from build123d import *

# Parameters (mm, degrees)
CROQUIS1_W               = 63
CROQUIS1_H               = 63
CROQUIS1_R               = 2
CROQUIS1_R_2             = 1.5
CROQUIS1_W_2             = 3
CROQUIS1_H_2             = 12
SALIENTE_EXTRUIR1_DEPTH  = 3
CROQUIS2_W               = 63
CROQUIS2_H               = 63
CROQUIS2_W_2             = 57
CROQUIS2_H_2             = 57
SALIENTE_EXTRUIR2_DEPTH  = 36
CROQUIS4_W               = 25
CROQUIS4_H               = 17
CORTAR_EXTRUIR2_DEPTH    = 60
SALIENTE_EXTRUIR8_DEPTH  = 60
CROQUIS8_W               = 3
CROQUIS8_H               = 12
CORTAR_EXTRUIR4_DEPTH    = 63
CROQUIS10_R              = 3
SALIENTE_EXTRUIR6_DEPTH  = 20
CROQUIS11_R              = 1.45
CORTAR_EXTRUIR6_DEPTH    = 9
REDONDEO1_R              = 2
CROQUIS13_W              = 25
CROQUIS13_H              = 25
CORTAR_EXTRUIR7_DEPTH    = 3
CROQUIS14_W              = 12
CROQUIS14_H              = 20
CORTAR_EXTRUIR8_DEPTH    = 5
CROQUIS15_R              = 3
SALIENTE_EXTRUIR9_DEPTH  = 20
CROQUIS16_W              = 15
CROQUIS16_H              = 18
SALIENTE_EXTRUIR10_DEPTH = 8
CROQUIS17_R              = 1.45
CORTAR_EXTRUIR9_DEPTH    = 20
CROQUIS18_W              = 3
CROQUIS18_H              = 12
SALIENTE_EXTRUIR11_DEPTH = 3
CROQUIS19_W              = 3
CROQUIS19_H              = 12
SALIENTE_EXTRUIR12_DEPTH = 3
REDONDEO3_R              = 1
CROQUIS20_R              = 3.125
CROQUIS20_R_2            = 2.625
CORTAR_EXTRUIR10_DEPTH   = 3
CROQUIS21_W              = 18.835847929
CROQUIS21_H              = 19.895765468
CORTAR_EXTRUIR11_DEPTH   = 18
CROQUIS22_R              = 1.45
SALIENTE_EXTRUIR13_DEPTH = 3
CROQUIS23_W              = 29
CROQUIS23_H              = 16
CORTAR_EXTRUIR12_DEPTH   = 6
CROQUIS24_W              = 3
CROQUIS24_H              = 5.5
CORTAR_EXTRUIR13_DEPTH   = 6
CROQUIS25_W              = 3
CROQUIS25_H              = 5.5
CORTAR_EXTRUIR14_DEPTH   = 30
CROQUIS26_W              = 25
CROQUIS26_H              = 0.5
CORTAR_EXTRUIR15_DEPTH   = 60
CROQUIS28_W              = 12
CROQUIS28_H              = 4
CORTAR_EXTRUIR16_DEPTH   = 6
SALIENTE_EXTRUIR14_DEPTH = 4.6
SALIENTE_EXTRUIR15_DEPTH = 1.5
REDONDEO4_R              = 2
CROQUIS31_W              = 2
CROQUIS31_H              = 3
CORTAR_EXTRUIR17_DEPTH   = 2


with BuildPart() as part:
    # Croquis1 → Saliente-Extruir1 (new body)
    with BuildSketch(Plane.XY):
        with Locations((31.5, 31.5)):
            Rectangle(CROQUIS1_W, CROQUIS1_H)
        with Locations((12, 57)):
            Circle(CROQUIS1_R, mode=Mode.SUBTRACT)
        with Locations((51, 57)):
            Circle(CROQUIS1_R, mode=Mode.SUBTRACT)
        with Locations((14.5, 5.5)):
            Circle(CROQUIS1_R_2, mode=Mode.SUBTRACT)
        with Locations((14.5, 23.5)):
            Circle(CROQUIS1_R_2, mode=Mode.SUBTRACT)
        with Locations((48.5, 5.5)):
            Circle(CROQUIS1_R_2, mode=Mode.SUBTRACT)
        with Locations((48.5, 23.5)):
            Circle(CROQUIS1_R_2, mode=Mode.SUBTRACT)
        with Locations((24.5, 14.5)):
            Rectangle(CROQUIS1_W_2, CROQUIS1_H_2, mode=Mode.SUBTRACT)
        with Locations((38.5, 14.5)):
            Rectangle(CROQUIS1_W_2, CROQUIS1_H_2, mode=Mode.SUBTRACT)
    extrude(amount=SALIENTE_EXTRUIR1_DEPTH)

    # Croquis2 → Saliente-Extruir2 (add)
    with BuildSketch(Plane(origin=(0, 0, 0), x_dir=(-1, 0, 0), z_dir=(0, 0, -1))):
        with Locations((-31.5, 31.5)):
            Rectangle(CROQUIS2_W, CROQUIS2_H)
        with Locations((-31.5, 31.5)):
            Rectangle(CROQUIS2_W_2, CROQUIS2_H_2, mode=Mode.SUBTRACT)
    extrude(amount=SALIENTE_EXTRUIR2_DEPTH)

    # Croquis4 → Cortar-Extruir2 (cut)
    with BuildSketch(Plane(origin=(0, 63, 0), x_dir=(1, 0, 0), z_dir=(0, 1, 0))):
        with Locations((31.5, 7.5)):
            Rectangle(CROQUIS4_W, CROQUIS4_H)
    extrude(amount=-CORTAR_EXTRUIR2_DEPTH, mode=Mode.SUBTRACT)

    # Croquis12 → Saliente-Extruir8 (add)
    with BuildSketch(Plane(origin=(0, 63, 0), x_dir=(1, 0, 0), z_dir=(0, 1, 0))):
        Polygon((19, -1), (17, -1), (17, 18), (46, 18), (46, -1), (44, -1), (44, 16), (19, 16), align=None)
    extrude(amount=-SALIENTE_EXTRUIR8_DEPTH)

    # Croquis8 → Cortar-Extruir4 (cut)
    with BuildSketch(Plane.ZY):
        with Locations((-1.5, 14.5)):
            Rectangle(CROQUIS8_W, CROQUIS8_H)
    extrude(amount=-CORTAR_EXTRUIR4_DEPTH, mode=Mode.SUBTRACT)

    # Croquis10 → Saliente-Extruir6 (add)
    with BuildSketch(Plane(origin=(0, 0, -36), x_dir=(-1, 0, 0), z_dir=(0, 0, -1))):
        with Locations((-3, 3)):
            Circle(CROQUIS10_R)
        with Locations((-60, 3)):
            Circle(CROQUIS10_R)
    extrude(amount=-SALIENTE_EXTRUIR6_DEPTH)

    # Croquis11 → Cortar-Extruir6 (cut)
    with BuildSketch(Plane(origin=(0, 0, -36), x_dir=(-1, 0, 0), z_dir=(0, 0, -1))):
        with Locations((-60, 3)):
            Circle(CROQUIS11_R)
        with Locations((-3, 3)):
            Circle(CROQUIS11_R)
    extrude(amount=-CORTAR_EXTRUIR6_DEPTH, mode=Mode.SUBTRACT)

    # Redondeo1
    redondeo1_edges = [part.edges().sort_by_distance(p)[0] for p in [
        (63, 0, -16.5),
        (0, 0, -16.5),
    ]]
    fillet(redondeo1_edges, radius=REDONDEO1_R)

    # Croquis13 → Cortar-Extruir7 (cut)
    with BuildSketch(Plane(origin=(0, 0, -18), x_dir=(-1, 0, 0), z_dir=(0, 0, -1))):
        with Locations((-31.5, 15.5)):
            Rectangle(CROQUIS13_W, CROQUIS13_H)
    extrude(amount=-CORTAR_EXTRUIR7_DEPTH, mode=Mode.SUBTRACT)

    # Croquis14 → Cortar-Extruir8 (cut)
    with BuildSketch(Plane(origin=(0, 63, 0), x_dir=(1, 0, 0), z_dir=(0, 1, 0))):
        with Locations((52, 10)):
            Rectangle(CROQUIS14_W, CROQUIS14_H)
        with Locations((11, 10)):
            Rectangle(CROQUIS14_W, CROQUIS14_H)
    extrude(amount=-CORTAR_EXTRUIR8_DEPTH, mode=Mode.SUBTRACT)

    # Croquis15 → Saliente-Extruir9 (add)
    with BuildSketch(Plane(origin=(0, 63, 0), x_dir=(1, 0, 0), z_dir=(0, 1, 0))):
        with Locations((3, 0)):
            Circle(CROQUIS15_R)
        with Locations((60, 0)):
            Circle(CROQUIS15_R)
        with Locations(Location((31.5, 31, 0), (0, 0, 270))):
            Circle(CROQUIS15_R)
    extrude(amount=-SALIENTE_EXTRUIR9_DEPTH)

    # Croquis16 → Saliente-Extruir10 (add)
    with BuildSketch(Plane.XZ.offset(-60)):
        with Locations((31.5, -27)):
            Rectangle(CROQUIS16_W, CROQUIS16_H)
    extrude(amount=SALIENTE_EXTRUIR10_DEPTH)

    # Croquis17 → Cortar-Extruir9 (cut)
    with BuildSketch(Plane(origin=(0, 63, 0), x_dir=(1, 0, 0), z_dir=(0, 1, 0))):
        with Locations(Location((3, 0, 0), (0, 0, 270))):
            Circle(CROQUIS17_R)
        with Locations(Location((60, 0, 0), (0, 0, 270))):
            Circle(CROQUIS17_R)
        with Locations(Location((31.5, 31, 0), (0, 0, 270))):
            Circle(CROQUIS17_R)
    extrude(amount=-CORTAR_EXTRUIR9_DEPTH, mode=Mode.SUBTRACT)

    # Croquis18 → Saliente-Extruir11 (add)
    with BuildSketch(Plane(origin=(63, 0, 0), x_dir=(0, 0, -1), z_dir=(1, 0, 0))):
        with Locations((1.5, 14.5)):
            Rectangle(CROQUIS18_W, CROQUIS18_H)
    extrude(amount=-SALIENTE_EXTRUIR11_DEPTH)

    # Croquis19 → Saliente-Extruir12 (add)
    with BuildSketch(Plane.ZY):
        with Locations((-1.5, 14.5)):
            Rectangle(CROQUIS19_W, CROQUIS19_H)
    extrude(amount=-SALIENTE_EXTRUIR12_DEPTH)

    # Redondeo3
    redondeo3_edges = [part.edges().sort_by_distance(p)[0] for p in [
        (31.5, 28, -18),
        (44, 15.5, -18),
        (19, 15.5, -18),
        (46, 31.5, -18),
        (17, 31.5, -18),
        (39, 52, -27),
        (24, 52, -27),
        (39, 56, -36),
        (24, 56, -36),
        (31.5, 52, -36),
    ]]
    fillet(redondeo3_edges, radius=REDONDEO3_R - 0.0001)  # a hair under: the kernel refuses the full size

    # Croquis20 → Cortar-Extruir10 (cut)
    with BuildSketch(Plane.XZ):
        with Locations(Location((10, -4, 0), (0, 0, 270))):
            Circle(CROQUIS20_R)
        with Locations(Location((10, -14, 0), (0, 0, 270))):
            Circle(CROQUIS20_R_2)
    extrude(amount=-CORTAR_EXTRUIR10_DEPTH, mode=Mode.SUBTRACT)

    # Croquis21 → Cortar-Extruir11 (cut)
    with BuildSketch(Plane(origin=(0, 0, -36), x_dir=(-1, 0, 0), z_dir=(0, 0, -1))):
        with Locations((-31.895496214, 50.052117266)):
            Rectangle(CROQUIS21_W, CROQUIS21_H)
    extrude(amount=-CORTAR_EXTRUIR11_DEPTH, mode=Mode.SUBTRACT)

    # Croquis22 → Saliente-Extruir13 (add)
    with BuildSketch(Plane(origin=(0, 63, 0), x_dir=(1, 0, 0), z_dir=(0, 1, 0))):
        with Locations((31.5, 31)):
            Circle(CROQUIS22_R)
    extrude(amount=-SALIENTE_EXTRUIR13_DEPTH)

    # Croquis23 → Cortar-Extruir12 (cut)
    with BuildSketch(Plane(origin=(0, 63, 0), x_dir=(1, 0, 0), z_dir=(0, 1, 0))):
        with Locations((31.5, 8)):
            Rectangle(CROQUIS23_W, CROQUIS23_H)
    extrude(amount=-CORTAR_EXTRUIR12_DEPTH, mode=Mode.SUBTRACT)

    # Croquis24 → Cortar-Extruir13 (cut)
    with BuildSketch(Plane(origin=(0, 0, 1), x_dir=(-1, 0, 0), z_dir=(0, 0, -1))):
        with Locations((-38.5, 5.75)):
            Rectangle(CROQUIS24_W, CROQUIS24_H)
        with Locations((-24.5, 5.75)):
            Rectangle(CROQUIS24_W, CROQUIS24_H)
    extrude(amount=-CORTAR_EXTRUIR13_DEPTH, mode=Mode.SUBTRACT)

    # Croquis25 → Cortar-Extruir14 (cut)
    with BuildSketch(Plane(origin=(46, 0, 0), x_dir=(0, 0, -1), z_dir=(1, 0, 0))):
        with Locations((1.5, 5.75)):
            Rectangle(CROQUIS25_W, CROQUIS25_H)
    extrude(amount=-CORTAR_EXTRUIR14_DEPTH, mode=Mode.SUBTRACT)

    # Croquis26 → Cortar-Extruir15 (cut)
    with BuildSketch(Plane(origin=(0, 63, 0), x_dir=(1, 0, 0), z_dir=(0, 1, 0))):
        with Locations((31.5, 16.25)):
            Rectangle(CROQUIS26_W, CROQUIS26_H)
    extrude(amount=-CORTAR_EXTRUIR15_DEPTH, mode=Mode.SUBTRACT)

    # Croquis28 → Cortar-Extruir16 (cut)
    with BuildSketch(Plane(origin=(0, 63, 0), x_dir=(1, 0, 0), z_dir=(0, 1, 0))):
        with Locations((11, 22)):
            Rectangle(CROQUIS28_W, CROQUIS28_H)
        with Locations((52, 22)):
            Rectangle(CROQUIS28_W, CROQUIS28_H)
    extrude(amount=-CORTAR_EXTRUIR16_DEPTH, mode=Mode.SUBTRACT)

    # Croquis29 → Saliente-Extruir14 (add)
    with BuildSketch(Plane.ZY):
        Polygon((-36, 10), (-15, 10), (-15, 12), (-15, 47), (-17, 47), (-17, 12), (-34, 12), (-34, 47), (-36, 47), (-36, 12), align=None)
    extrude(amount=SALIENTE_EXTRUIR14_DEPTH)

    # Croquis30 → Saliente-Extruir15 (add)
    with BuildSketch(Plane.ZY.offset(4.6)):
        Polygon((-36, 10), (-15, 10), (-15, 14), (-15, 47), (-19, 47), (-19, 14), (-32, 14), (-32, 47), (-36, 47), (-36, 14), align=None)
    extrude(amount=SALIENTE_EXTRUIR15_DEPTH)

    # Redondeo4
    redondeo4_edges = [part.edges().sort_by_distance(p)[0] for p in [
        (-3.05, 10, -36),
        (-3.05, 10, -15),
        (-6.1, 28.5, -36),
        (-6.1, 10, -25.5),
        (-6.1, 28.5, -15),
    ]]
    fillet(redondeo4_edges, radius=REDONDEO4_R)

    # Croquis31 → Cortar-Extruir17 (cut)
    with BuildSketch(Plane.ZY.offset(6.1)):
        with Locations((-33, 45.5)):
            Rectangle(CROQUIS31_W, CROQUIS31_H)
    extrude(amount=-CORTAR_EXTRUIR17_DEPTH, mode=Mode.SUBTRACT)


solid = part.part
Read the model definition and answer for the solid it produces. Units are mm, in the model's axes. A direction names the side the tool comes from. Round coordinates to 2 decimals unless told otherwise and drop trailing zeros. Loops run counter-clockwise (first coordinate to the right, second up) from the corner with the lowest first, then second, coordinate; pieces in that order, holes last.
Q1. Section B-B on z = -4 is taken. Write down the section's boundary in (x, y) (3 decimals).
Q2. Consider probe 1 along X at (y, z) = (26, -5); probe 2 along Z at (x, y) = (29, 56.5); probe 3 along Y at (x, z) = (28.5, -19.5). Determine where each line is inside the solid, lowest interval first.
Q3. Determine the mould class of faces 4 (the face through (18, 12, -3)), 5 (the face through (63, 33, -16)), 6 (the face through (2, 32, -36)) for opening direction Z: released by +Z, released by -Z, zero draft, split by the parting line, or undercut.
Q4. Section D-D on z = -30 is taken. Write down the section's boundary in (x, y).
Q5. Section A-A on x = 51 is taken. Write down the section's boundary in (y, z), and give its area (3 significant figures).
Q6. Each of these flat-tipped pins is pushed along its axis until it touches: pin 1 (1.6 mm diameter, centred on x = -3, z = -35.5, fed in from +Y); pin 2 (2 mm diameter, centred on x = -2.5, y = 33.5, fed in from +Z); pin 3 (1.5 mm diameter, centred on y = 12, z = -10, fed in from -X). Where does it stop, or does it pass through?
Q7. Section C-C on y = 8.5 is taken. Give the number of separate pieces and of enclosed holes in the cut face, and give its area (3 significant figures).
Q8. Which of the six approach directions +Z, -Z, +X, -X, +Y, -Y give full straight-line access (tool end or side, diameter ignored) to faces 1 (the face through (4.45, 3.06, -31.56)), 2 (the face through (11, 33, 0)), 3 (the face through (58.584, 53.14, -0.314))?
Output:
1. outline: (0, 2) arc R2 ccw to (2, 0) - (6.875, 0) - (6.875, 3) - (3, 3) - (3, 60) - (5, 60) - (5, 63) - (0, 63) - close; (13.125, 0) - (61, 0) arc R2 ccw to (63, 2) - (63, 63) - (58, 63) - (58, 60) - (60, 60) - (60, 3) - (46, 3) - (46, 57) - (44, 57) - (44, 3) - (19, 3) - (19, 57) - (17, 57) - (17, 3) - (13.125, 3) - close
2. probe 1: x = 0 to 3, 17 to 19, 44 to 46, 60 to 63
2. probe 2: z = -18 to -16.5, 1 to 3
2. probe 3: y = 0 to 3, 60 to 63
3. face 4: undercut
3. face 5: zero draft
3. face 6: released by -Z
4. outline: (-6.1, 12) arc R2 ccw to (-4.1, 10) - (0, 10) - (0, 2) arc R2 ccw to (2, 0) - (61, 0) arc R2 ccw to (63, 2) - (63, 63) - (0, 63) - (0, 12) - (-4.6, 12) - (-4.6, 14) - (-6.1, 14) - close; hole circle Ø2.9 at (3, 3); hole (3, 6) arc R3 cw to (6, 3) - (57, 3) arc R3 cw to (60, 6) - (60, 60) - (3, 60) - close; hole circle Ø2.9 at (60, 3)
5. outline: (0, -36) - (3, -36) - (3, 0) - (55, 0) - (55, 3) - (0, 3) - close; (59, 0) - (63, 0) - (63, 3) - (59, 3) - close; (60, -36) - (63, -36) - (63, -24) - (60, -24) - close
5. area: 321 mm2
6. pin 1: stops at y = 47
6. pin 2: stops at z = -15
6. pin 3: stops at x = 0
7. separate pieces: 5
7. enclosed holes: 0
7. area: 427 mm2
8. face 1: -Z
8. face 2: none
8. face 3: +Y
